Could you check a few things on this model? Use its own coordinates, in mm. A direction names the side the tool comes from. Round coordinates to 2 decimals unless told otherwise and drop trailing zeros. Loops run counter-clockwise (first coordinate to the right, second up) from the corner with the lowest first, then second, coordinate; pieces in that order, holes last. Notation, with made-up numbers: (88.5, 22) -> (131.5, 22) arc R20 ccw to (131.5, 55) -> close; hole circle Ø5 at (16, 75.5). An arc over 180 degrees is marked (long way). Write each question's results on one line, items separated by ' | '. Start each with the question number.
1) For P1, Ø2, axis at y = 5.5, z = -11.5, coming from the +X side; P2, Ø10, axis at y = 9.5, z = -1.5, coming from the -X side, each with a flat end and sliding along its axis, tell me the tip position at first contact or that it passes through.
2) Imagine slicing it at B-B, the plane y = 0. List the corners of the cut face in (x, z) for me (3 decimals), plus the area to 3 significant figures.
3) We'd pull the mould along Y, two halves only. Please class faces 1 (the flat face through (-55, 0, -18.415)), 2 (the cylindrical face through (-53.425, 2.026, -22.278)), 3 (the cylindrical face through (51.96, 4.56, -22.28)), 4 (the flat face through (0, 12.7, 16)): pulls with the +Y half, pulls with the -Y half, needs draft (parallel to the pull), parting line crosses it, or undercut.
4) Imagine slicing it at A-A, the plane z = -22. List the corners of the cut face in (x, y) for me, plus the area to 3 significant figures.
5) If I drill on probe 1 along Y at (x, z) = (-46.99, -24.25); probe 2 along X at (y, z) = (-6.75, -13.5); probe 3 along X at (y, z) = (-1.75, -23), over which ranges is the centre line in solid material (lowest first)?
6) Which directions (+Z, -Z, +X, -X, +Y, -Y) give clear straight access to the entire face, cutting with the end or side of a thin tool? Please do faces 5 (the cylindrical face through (-22.136, -0.178, 13.841)), 6 (the flat face through (40, 0, -26.035)), 7 (the flat face through (55, 0, -18.415)), 8 (the flat face through (-30.48, 0, 5)), 9 (the flat face through (0, -12.7, 16)).
7) Imagine slicing it at D-D, the plane z = -1. List the corners of the cut face in (x, y) for me.
8) Imagine slicing it at C-C, the plane x = 46.99. List the corners of the cut face in (y, z) for me (3 decimals), plus the area to 3 significant figures.
from build123d import *

# Parameters (mm, degrees)
F0_W     = 127
F0_H     = 52.07
F1_DEPTH = 12.7
F2_W     = 45.72
F2_H     = 25.4
F3_DEPTH = 40.64
F4_R     = 2.54
F5_W     = 33.02
F5_H     = 25.4
F6_DEPTH = 44.45
F7_R     = 2.54
F8_D     = 13.49248


with BuildPart() as f1:
    # F0 (on Front) → F1 (new body, symmetric)
    with BuildSketch(Plane.XZ):
        Rectangle(F0_W, F0_H)
    extrude(amount=F1_DEPTH, both=True)

    # F2 (on face) → F3 (cut)
    with BuildSketch(Plane(origin=(0, 0, -26.035), x_dir=(1, 0, 0), z_dir=(0, 0, -1))):
        Rectangle(F2_W, F2_H)
    extrude(amount=-F3_DEPTH, mode=Mode.SUBTRACT)

    # F4
    f4_edges = [f1.edges().sort_by_distance(p)[0] for p in [
        (-22.86, 0, 14.605),
        (22.86, 0, 14.605),
    ]]
    fillet(f4_edges, radius=F4_R)

    # F5 (on face) → F6 (cut)
    with BuildSketch(Plane.XY.offset(26.035)):
        with Locations((-46.99, 0)):
            Rectangle(F5_W, F5_H)
        with Locations((46.99, 0)):
            Rectangle(F5_W, F5_H)
    extrude(amount=-F6_DEPTH, mode=Mode.SUBTRACT)

    # F7
    f7_edges = [f1.edges().sort_by_distance(p)[0] for p in [
        (-30.48, 0, -18.415),
        (30.48, 0, -18.415),
        (-22.86, 0, -26.035),
        (22.86, 0, -26.035),
    ]]
    fillet(f7_edges, radius=F7_R)

    # F8 (through all)
    with Locations(Plane.XY.offset(26.035)):
        with Locations((-46.99, 0), (46.99, 0)):
            Hole(F8_D / 2)


solid = f1.part
Checked values:
1) P1: x = 30.48 | P2: x = -30.48
2) outline: (-63.5, -26.035) -> (-53.736, -26.035) -> (-53.736, -18.415) -> (-63.5, -18.415) -> close; (-40.244, -26.035) -> (-25.4, -26.035) arc R2.54 ccw to (-22.86, -23.495) -> (-22.86, 12.065) arc R2.54 cw to (-20.32, 14.605) -> (20.32, 14.605) arc R2.54 cw to (22.86, 12.065) -> (22.86, -23.495) arc R2.54 ccw to (25.4, -26.035) -> (40.244, -26.035) -> (40.244, -18.415) -> (33.02, -18.415) arc R2.54 cw to (30.48, -15.875) -> (30.48, 26.035) -> (-30.48, 26.035) -> (-30.48, -15.875) arc R2.54 cw to (-33.02, -18.415) -> (-40.244, -18.415) -> close; (53.736, -26.035) -> (63.5, -26.035) -> (63.5, -18.415) -> (53.736, -18.415) -> close | area: 1,620 mm^2
3) face 1: needs draft | face 2: undercut | face 3: undercut | face 4: pulls with the +Y half
4) outline: (-63.5, -12.7) -> (-22.86, -12.7) -> (-22.86, 12.7) -> (-63.5, 12.7) -> close; (22.86, -12.7) -> (63.5, -12.7) -> (63.5, 12.7) -> (22.86, 12.7) -> close; hole circle Ø13.49 at (-46.99, 0); hole circle Ø13.49 at (46.99, 0) | area: 1,780 mm^2
5) probe 1: -12.7 to -6.75, 6.75 to 12.7 | probe 2: -30.48 to -22.86, 22.86 to 30.48 | probe 3: -63.5 to -53.51, -40.47 to -22.86, 22.86 to 40.47, 53.51 to 63.5
6) face 5: -Z, +Y, -Y | face 6: -Z, +X, -X, +Y, -Y | face 7: +Z, +X, +Y, -Y | face 8: +Z, -X, +Y, -Y | face 9: +Z, -Z, +X, -X, -Y
7) outline: (-30.48, -12.7) -> (-22.86, -12.7) -> (-22.86, 12.7) -> (-30.48, 12.7) -> close; (22.86, -12.7) -> (30.48, -12.7) -> (30.48, 12.7) -> (22.86, 12.7) -> close
8) outline: (-12.7, -26.035) -> (-6.746, -26.035) -> (-6.746, -18.415) -> (-12.7, -18.415) -> close; (6.746, -26.035) -> (12.7, -26.035) -> (12.7, -18.415) -> (6.746, -18.415) -> close | area: 90.7 mm^2
